Model file for the job. Use its own axes, mm. Face numbers are marked on the shaded views. A direction names the side the tool comes from. Round coordinates to 2 decimals unless told otherwise and drop trailing zeros. Order: outer loops, then holes, each group sorted by start corner. A loop starts at its lowest first (then second) coordinate and runs counter-clockwise, first axis right, second up. Notation, with made-up numbers: (-9.5, -12.5) - (45.5, -12.5) arc R24 ccw to (45.5, 6.5) - close; hole circle Ø5 at (-18, 68). An arc over 180 degrees is marked (long way). Use one line per item in the form item = value.
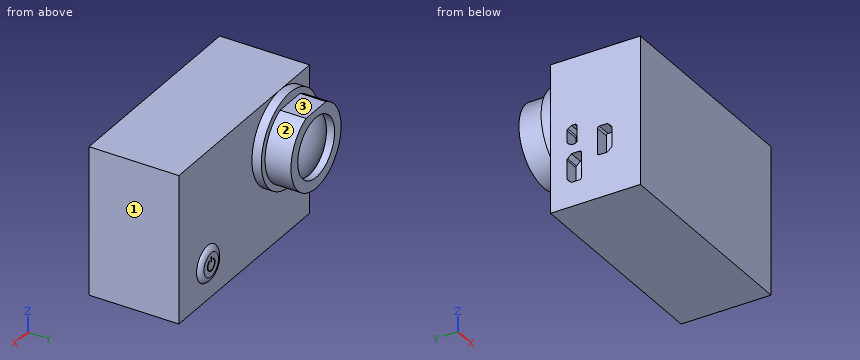
from build123d import *
from build123d.topology import SkipClean

# Parameters (mm, degrees)
CROQUIS1_W              = 59
CROQUIS1_H              = 41.21
SALIENTE_EXTRUIR1_DEPTH = 25
CROQUIS2_R              = 13
SALIENTE_EXTRUIR2_DEPTH = 9.81
CORTAR_EXTRUIR1_START   = -7.2
CROQUIS4_R              = 13
CROQUIS4_R_2            = 11.32
CORTAR_EXTRUIR1_DEPTH   = 7.2
CORTAR_EXTRUIR2_START   = -7.2
CORTAR_EXTRUIR2_DEPTH   = 7.2
CROQUIS7_R              = 8.32
CORTAR_EXTRUIR3_DEPTH   = 5
CROQUIS10_R             = 5
SALIENTE_EXTRUIR3_DEPTH = 1
REDONDEO1_R             = 2
CORTAR_EXTRUIR5_DEPTH   = 0.2
CROQUIS13_R             = 2.5
CORTAR_EXTRUIR6_DEPTH   = 5.2
ROSCA1_PITCH            = 0.8
CORTAR_EXTRUIR8_DEPTH   = 4
CROQUIS17_W             = 9.488888662
CROQUIS17_H             = 7.855040283
SALIENTE_EXTRUIR4_DEPTH = 10


with BuildPart() as part:
    # Croquis1 → Saliente-Extruir1 (new body)
    with BuildSketch(Plane(origin=(0, 0, 0), x_dir=(1, 0, 0), z_dir=(0, 1, 0))):
        Rectangle(CROQUIS1_W, CROQUIS1_H)
    extrude(amount=SALIENTE_EXTRUIR1_DEPTH)

    # Croquis2 → Saliente-Extruir2 (add)
    with BuildSketch(Plane(origin=(0, 25, 0), x_dir=(1, 0, 0), z_dir=(0, 1, 0))):
        with Locations(Location((-16.5, -7.605, 0), (0, 0, 270))):
            Circle(CROQUIS2_R)
    extrude(amount=SALIENTE_EXTRUIR2_DEPTH)

    # Croquis4 → Cortar-Extruir1 (cut)
    with BuildSketch(Plane(origin=(0, 34.81, 0), x_dir=(1, 0, 0), z_dir=(0, 1, 0)).offset(CORTAR_EXTRUIR1_START)):
        with Locations(Location((-16.5, -7.605, 0), (0, 0, 270))):
            Circle(CROQUIS4_R)
        with Locations(Location((-16.5, -7.605, 0), (0, 0, 270))):
            Circle(CROQUIS4_R_2, mode=Mode.SUBTRACT)
    extrude(amount=CORTAR_EXTRUIR1_DEPTH, mode=Mode.SUBTRACT)

    # Croquis6 → Cortar-Extruir2 (cut)
    with BuildSketch(Plane(origin=(0, 34.81, 0), x_dir=(1, 0, 0), z_dir=(0, 1, 0)).offset(CORTAR_EXTRUIR2_START)):
        with BuildLine():
            Line((-12.00663823, -17.995), (-20.99336177, -17.995))
            ThreePointArc((-20.99336177, -17.995), (-16.5, -18.925), (-12.00663823, -17.995))
        make_face()
    extrude(amount=CORTAR_EXTRUIR2_DEPTH, mode=Mode.SUBTRACT)

    # Croquis7 → Cortar-Extruir3 (cut)
    with BuildSketch(Plane(origin=(0, 34.81, 0), x_dir=(1, 0, 0), z_dir=(0, 1, 0))):
        with Locations(Location((-16.568588437, -7.600561682, 0), (0, 0, 270))):
            Circle(CROQUIS7_R)
    extrude(amount=-CORTAR_EXTRUIR3_DEPTH, mode=Mode.SUBTRACT)

    # Croquis9 → Revolución2 (revolve)
    with BuildSketch(Plane.ZY.offset(16.5)):
        with BuildLine():
            Line((15.920561682, 32.31), (7.14, 32.31))
            Line((7.14, 32.31), (7.14, 34.81))
            ThreePointArc((7.14, 34.81), (11.704763506, 34.17282232), (15.920561682, 32.31))
        make_face()
    revolve(axis=Axis((-16.5, 32.31, 7.14), (0, 1, 0)))

    # Croquis10 → Saliente-Extruir3 (add)
    with BuildSketch(Plane(origin=(0, 25, 0), x_dir=(1, 0, 0), z_dir=(0, 1, 0))):
        with Locations(Location((16.5, 10.605, 0), (0, 0, 270))):
            Circle(CROQUIS10_R)
    extrude(amount=SALIENTE_EXTRUIR3_DEPTH)

    # Redondeo1
    # the kernel refuses this fillet: 2 mm, written as the material it takes off along each edge
    with BuildSketch(Plane(origin=(16.5, 26, -10.605), x_dir=(0, 0, 1), z_dir=(-1, 0, 0))) as redondeo1_piece_1:
        with BuildLine():
            CenterArc((3.267949192, -2), REDONDEO1_R, 30, 60)
            Line((3.267949192, 0), (3.267949192, 0.04))
            Line((3.267949192, 0.04), (5, 0.04))
            Line((5, 0.04), (5.04, 0))
            ThreePointArc((5.04, 0), (5.04, -0.5), (5.034641016, -0.98))
            Line((5.034641016, -0.98), (5, -1))
        make_face()
    revolve(axis=Axis((16.5, 26, -10.605), (0, 1, 0)), mode=Mode.SUBTRACT)

    # Croquis12 → Cortar-Extruir5 (cut)
    with BuildSketch(Plane(origin=(0, 26, 0), x_dir=(1, 0, 0), z_dir=(0, 1, 0))):
        with BuildLine():
            Line((15.693774225, 9.194547086), (15.693774225, 9.312956107))
            ThreePointArc((15.693774225, 9.312956107), (15.687825385, 9.33660976), (15.671394411, 9.354634942))
            ThreePointArc((15.671394411, 9.354634942), (16.5, 12.105), (17.328605589, 9.354634942))
            ThreePointArc((17.328605589, 9.354634942), (17.312174615, 9.33660976), (17.306225775, 9.312956107))
            Line((17.306225775, 9.312956107), (17.306225775, 9.194547086))
            ThreePointArc((17.306225775, 9.194547086), (17.331703456, 9.150973517), (17.38217201, 9.151806089))
            ThreePointArc((17.38217201, 9.151806089), (16.5, 12.305), (15.61782799, 9.151806089))
            ThreePointArc((15.61782799, 9.151806089), (15.668296544, 9.150973517), (15.693774225, 9.194547086))
        make_face()
        with BuildLine():
            Line((16.55, 8.355), (16.45, 8.355))
            ThreePointArc((16.45, 8.355), (16.414644661, 8.369644661), (16.4, 8.405))
            Line((16.4, 8.405), (16.4, 9.805))
            ThreePointArc((16.4, 9.805), (16.414644661, 9.840355339), (16.45, 9.855))
            Line((16.45, 9.855), (16.55, 9.855))
            ThreePointArc((16.55, 9.855), (16.585355339, 9.840355339), (16.6, 9.805))
            Line((16.6, 9.805), (16.6, 8.405))
            ThreePointArc((16.6, 8.405), (16.585355339, 8.369644661), (16.55, 8.355))
        make_face()
    extrude(amount=-CORTAR_EXTRUIR5_DEPTH, mode=Mode.SUBTRACT)

    # Croquis13 → Cortar-Extruir6 (cut)
    with BuildSketch(Plane(origin=(0, 0, -20.605), x_dir=(-1, 0, 0), z_dir=(0, 0, -1))):
        with Locations((19, 13.3)):
            Circle(CROQUIS13_R)
    extrude(amount=-CORTAR_EXTRUIR6_DEPTH, mode=Mode.SUBTRACT)

    # Rosca1: the profile of Perfil de rosca1 profile screwed along a right-hand helix of 6.5 turns, 8 arcs to a turn; built about Z, then put on its axis
    with SkipClean():  # the faces are left unmerged after this step: merging them gives an invalid solid
        rosca1_z = Axis((0, 0, 0), (0, 0, 1))
        rosca1_corners = [(2.5003, 0, -0.000173205), (2.5003, 0, 0.700173203), (2.0669873, 0, 0.449999999), (2.0669873, 0, 0.249999999)]
        with BuildLine(mode=Mode.PRIVATE) as rosca1_profile:
            Line(rosca1_corners[0], rosca1_corners[1])
            Line(rosca1_corners[1], rosca1_corners[2])
            Line(rosca1_corners[2], rosca1_corners[3])
            Line(rosca1_corners[3], rosca1_corners[0])
        rosca1_cap = Face(rosca1_profile.wire())
        rosca1_turn_angles = [0, 22.5, 45, 67.5, 90, 112.5, 135, 157.5, 180, 202.5, 225, 247.5, 270, 292.5, 315, 337.5, 360]
        rosca1_turn_weights = [1, 0.9238795325112867, 1, 0.9238795325112867, 1, 0.9238795325112867, 1, 0.9238795325112867, 1, 0.9238795325112867, 1, 0.9238795325112867, 1, 0.9238795325112867, 1, 0.9238795325112867, 1]
        rosca1_turn_rails = [Edge.make_bspline([Vector(p[0], p[1], 0).rotate(rosca1_z, rosca1_turn_angles[k]) / rosca1_turn_weights[k] + Vector(0, 0, p[2] + ROSCA1_PITCH * rosca1_turn_angles[k] / 360) for k in range(17)], [0, 0, 0, 1, 1, 2, 2, 3, 3, 4, 4, 5, 5, 6, 6, 7, 7, 8, 8, 8], 2, rosca1_turn_weights) for p in rosca1_corners]
        rosca1_turn_sides = [Face.make_surface_from_curves(rosca1_turn_rails[p[0]], rosca1_turn_rails[p[1]]) for p in [(0, 1), (1, 2), (2, 3), (3, 0)]]
        rosca1_last_angles = [2160, 2182.5, 2205, 2227.5, 2250, 2272.5, 2295, 2317.5, 2340]
        rosca1_last_weights = [1, 0.9238795325112867, 1, 0.9238795325112867, 1, 0.9238795325112867, 1, 0.9238795325112867, 1]
        rosca1_last_rails = [Edge.make_bspline([Vector(p[0], p[1], 0).rotate(rosca1_z, rosca1_last_angles[k]) / rosca1_last_weights[k] + Vector(0, 0, p[2] + ROSCA1_PITCH * rosca1_last_angles[k] / 360) for k in range(9)], [0, 0, 0, 1, 1, 2, 2, 3, 3, 4, 4, 4], 2, rosca1_last_weights) for p in rosca1_corners]
        rosca1_last_sides = [Face.make_surface_from_curves(rosca1_last_rails[p[0]], rosca1_last_rails[p[1]]) for p in [(0, 1), (1, 2), (2, 3), (3, 0)]]
        rosca1 = Plane(origin=(-19, 13.3, -20.605), x_dir=(1, 0, 0), z_dir=(0, 0, 1)) * Solid(Shell([*[p.moved(Location((0, 0, ROSCA1_PITCH * i))) for i in range(6) for p in rosca1_turn_sides], *rosca1_last_sides, rosca1_cap, rosca1_cap.rotate(rosca1_z, 2340).moved(Location((0, 0, ROSCA1_PITCH * 2340 / 360)))]))
        add(rosca1)

    # Croquis16 → Cortar-Extruir8 (cut)
    with SkipClean():  # the faces are left unmerged after this step: merging them gives an invalid solid
        with BuildSketch(Plane.ZY.offset(29.5)):
            with BuildLine():
                Line((-5.945, 19.16), (-6.951704527, 20.240791007))
                ThreePointArc((-6.951704527, 20.240791007), (-7.118070383, 20.358473284), (-7.317575391, 20.4))
                Line((-7.317575391, 20.4), (-12.532424609, 20.4))
                ThreePointArc((-12.532424609, 20.4), (-12.731929617, 20.358473284), (-12.898295473, 20.240791007))
                Line((-12.898295473, 20.240791007), (-13.905, 19.16))
                Line((-13.905, 19.16), (-13.905, 16.9))
                ThreePointArc((-13.905, 16.9), (-13.758553391, 16.546446609), (-13.405, 16.4))
                Line((-13.405, 16.4), (-6.445, 16.4))
                ThreePointArc((-6.445, 16.4), (-6.091446609, 16.546446609), (-5.945, 16.9))
                Line((-5.945, 16.9), (-5.945, 19.16))
            make_face()
            with BuildLine():
                Line((1.93, 19.16), (1.330694375, 20.15750198))
                ThreePointArc((1.330694375, 20.15750198), (1.148320916, 20.335172948), (0.902100476, 20.4))
                Line((0.902100476, 20.4), (-2.392100476, 20.4))
                ThreePointArc((-2.392100476, 20.4), (-2.638320916, 20.335172948), (-2.820694375, 20.15750198))
                Line((-2.820694375, 20.15750198), (-3.42, 19.16))
                Line((-3.42, 19.16), (-3.42, 18.16))
                ThreePointArc((-3.42, 18.16), (-3.273553391, 17.806446609), (-2.92, 17.66))
                Line((-2.92, 17.66), (1.43, 17.66))
                ThreePointArc((1.43, 17.66), (1.783553391, 17.806446609), (1.93, 18.16))
                Line((1.93, 18.16), (1.93, 19.16))
            make_face()
            with BuildLine():
                ThreePointArc((-1.736855309, 8.079208993), (-1.903221166, 7.961526716), (-2.102726174, 7.92))
                Line((-2.102726174, 7.92), (-7.317575391, 7.92))
                ThreePointArc((-7.317575391, 7.92), (-7.517080399, 7.961526716), (-7.683446256, 8.079208993))
                Line((-7.683446256, 8.079208993), (-8.690150783, 9.16))
                Line((-8.690150783, 9.16), (-8.690150783, 11.42))
                ThreePointArc((-8.690150783, 11.42), (-8.543704173, 11.773553391), (-8.190150783, 11.92))
                Line((-8.190150783, 11.92), (-1.230150783, 11.92))
                ThreePointArc((-1.230150783, 11.92), (-0.876597392, 11.773553391), (-0.730150783, 11.42))
                Line((-0.730150783, 11.42), (-0.730150783, 9.16))
                Line((-0.730150783, 9.16), (-1.736855309, 8.079208993))
            make_face()
        extrude(amount=-CORTAR_EXTRUIR8_DEPTH, mode=Mode.SUBTRACT)

    # Croquis17 → Saliente-Extruir4 (add)
    with BuildSketch(Plane(origin=(0, 0, -20.605), x_dir=(-1, 0, 0), z_dir=(0, 0, -1))):
        with Locations((19.260558774, 13.137356389)):
            Rectangle(CROQUIS17_W, CROQUIS17_H)
    extrude(amount=-SALIENTE_EXTRUIR4_DEPTH)


solid = part.part
(1) Slice it at B-B on z = 3.5. Give the cut face in (x, y), then the cut area to 3 significant figures.
Report:
outline = (-29.5, 0) - (29.5, 0) - (29.5, 25) - (-4.17, 25) - (-4.17, 27.61) - (-5.95, 27.61) - (-5.95, 34.81) - (-9.33, 34.81) - (-9.33, 32.74) arc R16.27 ccw to (-23.81, 32.67) - (-23.81, 34.81) - (-27.05, 34.81) - (-27.05, 27.61) - (-28.83, 27.61) - (-28.83, 25) - (-29.5, 25) - close; hole (-23.81, 29.81) - (-9.33, 29.81) - (-9.33, 32.31) - (-23.81, 32.31) - close
area = 1,640 mm2
(2) Slice it at A-A on x = -9. Give the cut face in (y, z) (3 decimals), then the cut area to 3 significant figures.
Report:
outline = (0, -20.605) - (25, -20.605) - (25, -3.013) - (27.61, -3.013) - (27.61, -0.874) - (34.81, -0.874) - (34.81, 4.145) - (32.723, 4.145) arc R14.887 ccw to (32.503, 11.056) - (34.81, 11.056) - (34.81, 16.084) - (27.61, 16.084) - (27.61, 18.223) - (25, 18.223) - (25, 20.605) - (0, 20.605) - close; hole (29.81, 4.145) - (32.31, 4.145) - (32.31, 11.056) - (29.81, 11.056) - close
area = 1,180 mm2
(3) Pin check, flat tips, straight feed: pin 1 (5 mm diameter, centred on x = 15.5, z = 1, fed in from -Y); pin 2 (3.5 mm diameter, centred on x = -18, y = 29.5, fed in from +Z) (3 decimals); pin 3 (4 mm diameter, centred on x = 1, z = 12, fed in from +Y); pin 4 (12.5 mm diameter, centred on x = 11, z = -9.5, fed in from +Y). Stop position of each tip, or through.
Report:
pin_1 = 0
pin_2 = 17.995
pin_3 = 25
pin_4 = 26
(4) Probe probe 1 along Y at (x, z) = (-4, 12); probe 2 along Y at (x, z) = (-11.5, 13.5); probe 3 along Y at (x, z) = (-19.5, 13). List the from-to ranges inside material, lowest first. Write a range as [from, to].
Report:
probe_1 = [0, 25]
probe_2 = [0, 29.81], [32.31, 32.72]
probe_3 = [0, 29.81], [32.31, 33.45]
(5) Slice it at D-D on x = 25. Give the cut face in (y, z) (3 decimals).
Report:
outline = (0, -20.605) - (25, -20.605) - (25, 20.605) - (0, 20.605) - close
(6) Tool access for the marked faces 1, 2 and 3: list every direction of +Z, -Z, +X, -X, +Y, -Y with a clear straight run to the whole face (end or side of a thin tool).
Report:
face_1 = +Z, -Z, +X, +Y, -Y
face_2 = +Y
face_3 = +Z, +X, -X, +Y
(7) Slice it at C-C on z = 17. Give the cut face in (x, y), then the cut area to 3 significant figures.
Report:
outline = (-29.5, 0) - (29.5, 0) - (29.5, 25) - (-7.51, 25) - (-7.51, 27.61) - (-10.19, 27.61) - (-10.19, 34.81) - (-22.81, 34.81) - (-22.81, 27.61) - (-25.49, 27.61) - (-25.49, 25) - (-29.5, 25) - close
area = 1,610 mm2
